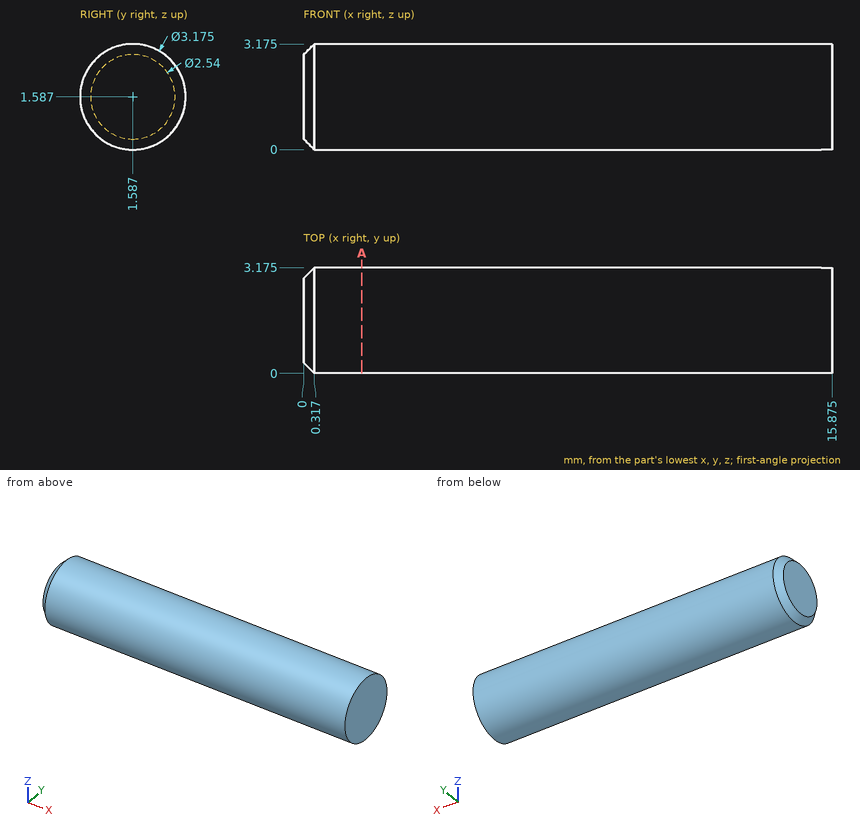
Source: three-view drawing plus pictorial views. Frame: mm from the lowest corner of the part. Round coordinates to 2 decimals unless told otherwise and drop trailing zeros. Loops run counter-clockwise (first coordinate to the right, second up) from the corner with the lowest first, then second, coordinate; pieces in that order, holes last.
Q1. Section A-A on x = 1.75. Return loops of the section in (y, z) (1 decimal).
Q2. Material intervals for L1, parallel to Z at x = 4.75, y = 1.7 (1 decimal); L2, parallel to Y at x = 4, z = 1.75; L3, parallel to X at y = 1.45, z = 0.2 (1 decimal), sorted ascending.
Q3. Pin query (flat end, axial travel): P1, Ø1, axis at x = 4, z = 0.5, coming from the +Y side. Return the tip coordinate at first contact, or that it passes through.
Evaluation:
1. outline: circle Ø3.2 at (1.6, 1.6)
2. L1: z = 0 to 3.2
2. L2: y = 0.01 to 3.17
2. L3: x = 0.1 to 15.9
3. P1: stops at y = 3.06
